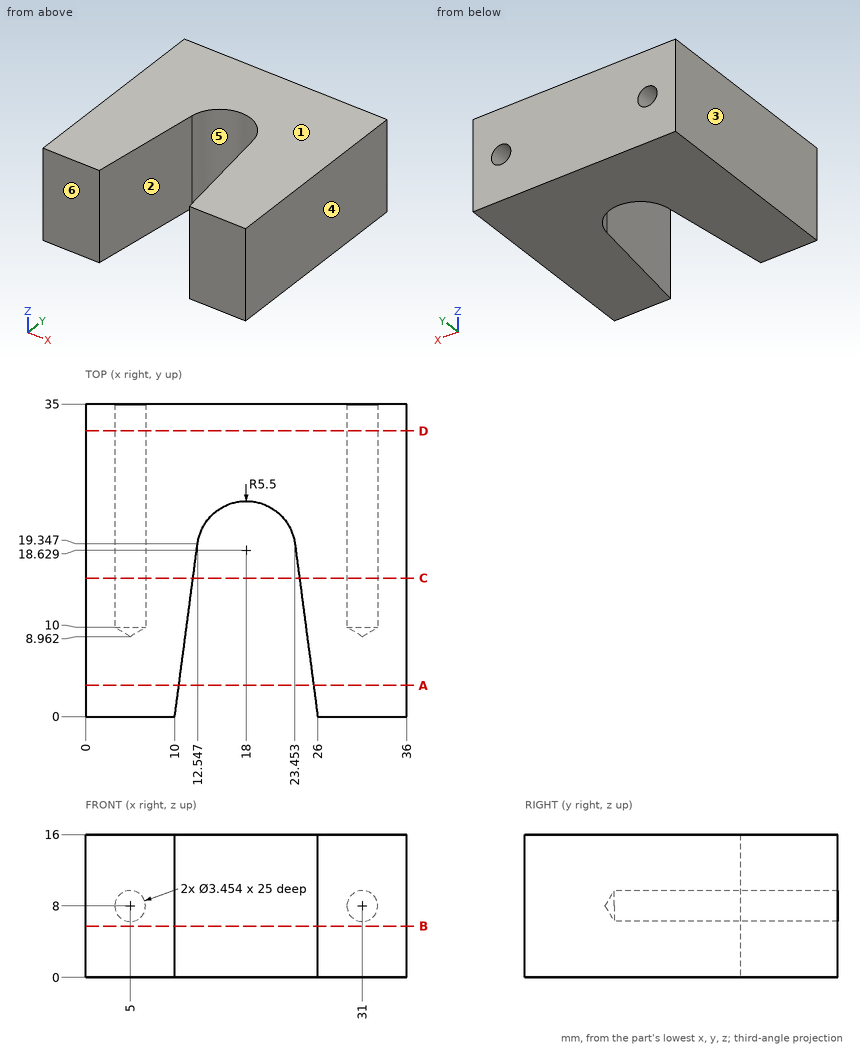
Geometry: see drawing. Coordinates: mm, zero at the bounding-box minimum. A direction names the side the tool comes from. Give positions to 0.01 mm unless a question says otherwise; leave off trailing zeros. Loops run counter-clockwise (first coordinate to the right, second up) from the corner with the lowest first, then second, coordinate; pieces in that order, holes last. Notation, with made-up numbers: M 27.25,-10 L 66.25,-10 A31 cw 66.25,14 Z; hole C 48,-36 d11. An arc over 180 degrees is marked long. Use one line per item in the form item = value.
1. Section query A-A, the plane y = 3.5. Return the cut outline in (x, z), and give its area (3 significant figures).
Numbers:
outline = M 0,0 L 10.46,0 L 10.46,16 L 0,16 Z; M 25.54,0 L 36,0 L 36,16 L 25.54,16 Z
area = 335 mm²
2. Pull-direction query (X, two-part tool) for the marked faces 3, 4, 5 and 6; classes: released by +X, released by -X, zero draft, split by the parting line, or undercut.
Numbers:
face_3 = released by -X
face_4 = released by +X
face_5 = undercut
face_6 = zero draft
3. Section query D-D, the plane y = 32. Return the cut outline in (x, z) (1 decimal).
Numbers:
outline = M 0,0 L 36,0 L 36,16 L 0,16 Z; hole C 5,8 d3.5; hole C 31,8 d3.5
4. Section query C-C, the plane y = 15.5. Return the cut outline in (x, z) (1 decimal).
Numbers:
outline = M 0,0 L 12,0 L 12,16 L 0,16 Z; M 24,0 L 36,0 L 36,16 L 24,16 Z; hole C 5,8 d3.5; hole C 31,8 d3.5
5. Reachability of the marked faces 1 and 2 from +Z, -Z, +X, -X, +Y, -Y: full face, straight path, thin tool, end or side. Return the list, or none.
Numbers:
face_1 = +Z, +X, -X, +Y, -Y
face_2 = +Z, -Z, -Y
6. Section query B-B, the plane z = 5.75. Return the cut outline in (x, y).
Numbers:
outline = M 0,0 L 10,0 L 12.55,19.35 A5.5 cw 23.45,19.35 L 26,0 L 36,0 L 36,35 L 0,35 Z
7. Line query: L1, parallel to X at y = 25.25, z = 8; L2, parallel to Z at x = 5, y = 29; L3, parallel to X at y = 20.5, z = 8.25. Output: solid intervals per line, ascending.
Numbers:
L1 = 0 to 3.27, 6.73 to 29.27, 32.73 to 36
L2 = 0 to 6.27, 9.73 to 16
L3 = 0 to 3.29, 6.71 to 12.83, 23.17 to 29.29, 32.71 to 36
